Source: CAD feature listing. Evaluate the final solid. Frame: model axes, mm. Give positions to 0.01 mm unless a question says otherwise; leave off trailing zeros. Order: outer loops, then holes, each group sorted by start corner. A loop starts at its lowest first (then second) coordinate and runs counter-clockwise, first axis right, second up. Notation, with made-up numbers: (-9.5, 24) -> (21.5, 24) arc R35 ccw to (21.5, 59) -> close; hole circle Ø11 at (68, 36). An arc over 180 degrees is marked (long way). Use CSV: the item, a comma, the result in double quotes.
```python
from build123d import *

# Parameters (mm, degrees)
SKETCH1_R           = 1.7
BOSS_EXTRUDE1_DEPTH = 3
FILLET1_R           = 1


with BuildPart() as part:
    # Sketch1 → Boss-Extrude1 (new body)
    with BuildSketch(Plane.XZ.offset(4)):
        with BuildLine():
            Line((-20, -25), (20, -25))
            ThreePointArc((20, -25), (23.535533906, -23.535533906), (25, -20))
            Line((25, -20), (25, 20))
            ThreePointArc((25, 20), (23.535533906, 23.535533906), (20, 25))
            Line((20, 25), (-20, 25))
            ThreePointArc((-20, 25), (-23.535533906, 23.535533906), (-25, 20))
            Line((-25, 20), (-25, -20))
            ThreePointArc((-25, -20), (-23.535533906, -23.535533906), (-20, -25))
        make_face()
        with Locations((-20, 20)):
            Circle(SKETCH1_R, mode=Mode.SUBTRACT)
        with Locations((20, 20)):
            Circle(SKETCH1_R, mode=Mode.SUBTRACT)
        with Locations((-20, -20)):
            Circle(SKETCH1_R, mode=Mode.SUBTRACT)
        with Locations((20, -20)):
            Circle(SKETCH1_R, mode=Mode.SUBTRACT)
    extrude(amount=BOSS_EXTRUDE1_DEPTH)

    # Fillet1
    fillet1_edges = [part.edges().sort_by_distance(p)[0] for p in [
        (23.535533906, -7, -23.535533906),
        (25, -7, 0),
        (23.535533906, -7, 23.535533906),
        (0, -7, 25),
        (-23.535533906, -7, 23.535533906),
        (-25, -7, 0),
        (-23.535533906, -7, -23.535533906),
        (0, -7, -25),
    ]]
    fillet(fillet1_edges, radius=FILLET1_R)


solid = part.part
```
1. Section query A-A on y = -4.7. Return loops of the section in (x, z), plus the area to 3 significant figures.
Answer below:
outline,"(-25, -20) arc R5 ccw to (-20, -25) -> (20, -25) arc R5 ccw to (25, -20) -> (25, 20) arc R5 ccw to (20, 25) -> (-20, 25) arc R5 ccw to (-25, 20) -> close; hole circle Ø3.4 at (-20, -20); hole circle Ø3.4 at (-20, 20); hole circle Ø3.4 at (20, -20); hole circle Ø3.4 at (20, 20)"
area,"2,440 mm²"
2. Mould query, pull axis X, two halves, no side actions, for faces 1 (the cylindrical face through (23, -5, -24)), 2 (the cylindrical face through (20.914, -5.479, -18.567)), 3 (the flat face through (0, -4, 0)). Classes: released by +X, released by -X, zero draft, split by the parting line, or undercut.
Answer below:
face 1,"released by +X"
face 2,"undercut"
face 3,"zero draft"
3. Ray query, line 1 along Z through (x, y) = (20, -5.1); line 2 along Z through (x, y) = (19, -5.35); line 3 along X through (y, z) = (-5.4, -21.5). Return the intervals inside material, ascending.
Answer below:
line 1,"z = -25 to -21.7, -18.3 to 18.3, 21.7 to 25"
line 2,"z = -25 to -21.37, -18.63 to 18.63, 21.37 to 25"
line 3,"x = -24.77 to -20.8, -19.2 to 19.2, 20.8 to 24.77"
4. Section query B-B on z = 21. Count the separate pieces of the cut face and the enclosed holes in it, plus the area to 3 significant figures.
Answer below:
separate pieces,"3"
enclosed holes,"0"
area,"132 mm²"
5. Pin query (flat end, axial travel): P1, Ø4, axis at x = -20, z = 20, coming from the +Y side. Return the tip coordinate at first contact, or that it passes through.
Answer below:
P1,"stops at y = -4"
